```python
from build123d import *

# Parameters (mm, degrees)
SKETCH_R              = 9.5
PAD_DEPTH             = 0.4
POLARPATTERN_COUNT    = 6
PAD001_DEPTH          = 25
POLARPATTERN001_COUNT = 6
SKETCH002_R           = 9.5
POCKET_DEPTH          = 2
POLARPATTERN002_COUNT = 6
SKETCH003_R           = 1.5
PAD002_DEPTH          = 25


with BuildPart() as part:
    # Sketch → Pad (new body, symmetric)
    with BuildSketch(Plane.XZ):
        with BuildLine():
            Line((0, 0), (57, 0))
            Line((57, 0), (57, 25))
            Line((57, 25), (0, 25))
            Line((0, 25), (0, 22))
            ThreePointArc((0, 3), (9.5, 12.5), (0, 22))
            Line((0, 3), (0, 0))
        make_face()
        with Locations((22, 12.5)):
            Circle(SKETCH_R, mode=Mode.SUBTRACT)
        with Locations((44, 12.5)):
            Circle(SKETCH_R, mode=Mode.SUBTRACT)
    pad = extrude(amount=PAD_DEPTH, both=True)

    # PolarPattern: Pad ×6 about axis
    polarpattern_axis = Axis((0, 0, 0), (0, 0, 1))
    for i in range(1, POLARPATTERN_COUNT):
        add(pad.rotate(polarpattern_axis, i * 360 / POLARPATTERN_COUNT))

    # Sketch001 (on Face55 of PolarPattern) → Pad001 (join)
    with BuildSketch(Plane(origin=(0, 0, 25), x_dir=(-1, 0, 0), z_dir=(0, 0, 1))):
        Polygon((-28.15359, 49.563448), (28.15359, 49.563448), (27.69171, 48.763448), (-27.69171, 48.763448), align=None)
    pad001 = extrude(amount=-PAD001_DEPTH)

    # PolarPattern001: Pad001 ×6 about axis
    polarpattern001_axis = Axis((0, 0, 25), (0, 0, 1))
    for i in range(1, POLARPATTERN001_COUNT):
        add(pad001.rotate(polarpattern001_axis, i * 360 / POLARPATTERN001_COUNT))

    # Sketch002 (on Face59 of Pad001) → Pocket (cut)
    with BuildSketch(Plane.XZ.offset(49.563448)):
        with Locations((-12.5, 12.5)):
            Circle(SKETCH002_R)
        with Locations((12.5, 12.5)):
            Circle(SKETCH002_R)
    pocket = extrude(amount=-POCKET_DEPTH, mode=Mode.SUBTRACT)

    # PolarPattern002: Pocket ×6 about axis
    polarpattern002_axis = Axis((0, 0, 0), (0, 0, 1))
    for i in range(1, POLARPATTERN002_COUNT):
        add(pocket.rotate(polarpattern002_axis, i * 360 / POLARPATTERN002_COUNT), mode=Mode.SUBTRACT)

    # Sketch003 (on Face81 of PolarPattern002) → Pad002 (join)
    with BuildSketch(Plane(origin=(0, 0, 25), x_dir=(-1, 0, 0), z_dir=(0, 0, 1))):
        Circle(SKETCH003_R)
    extrude(amount=-PAD002_DEPTH)


solid = part.part
```
Input: part model. Units: mm. Frame: model coordinates. A direction names the side the tool comes from. Give positions to 0.01 mm unless a question says otherwise; leave off trailing zeros. Return JSON: item names as keys, results as strings.
1) Line query: L1, parallel to Z at x = 44, y = 0; L2, parallel to Y at x = 1, z = 3.5; L3, parallel to Y at x = 27, z = 24. Output: solid intervals per line, ascending. Write a range as [from, to].
Taken from the geometry:
{"L1": "z = [0, 3], [22, 25]", "L2": "y = [-49.56, -48.76], [-1.12, 1.12], [48.76, 49.56]", "L3": "y = [-49.56, -48.76], [-47.57, -45.97], [-0.4, 0.4], [45.97, 47.57], [48.76, 49.56]"}
2) Section query A-A on x = -39. Count the separate pieces of the cut face and the enclosed holes in it, and give its area (3 significant figures).
Taken from the geometry:
{"separate pieces": "6", "enclosed holes": "0", "area": "36.9 mm2"}
3) Contact query for flat-ended pins moving along their axis: pin 1 (10 mm diameter, centred on y = 14, z = 6.5, fed in from +X); pin 2 (11.5 mm diameter, centred on x = 12.5, z = 12.5, fed in from -Y); pin 3 (10 mm diameter, centred on y = 23, z = 3.5, fed in from -X). Output: stop coordinate, or through.
Taken from the geometry:
{"pin 1": "stops at x = 51.82", "pin 2": "stops at y = -30.59", "pin 3": "stops at x = -46.84"}
4) Mould query, pull axis X, two halves, no side actions, for faces 1 (the face through (16.878, -30.033, 15.453)), 2 (the face through (-42.73, -25.12, 12.68)), 3 (the face through (0, 49.563, 13)). Classes: released by +X, released by -X, zero draft, split by the parting line, or undercut.
Taken from the geometry:
{"face 1": "undercut", "face 2": "released by -X", "face 3": "zero draft"}
5) Access query for faces 4 (the face through (9.5, 0.01, 12.69)), 5 (the face through (-5.5, 49.17, 18.92)), 6 (the face through (42.037, -24.717, 12.675)). Directions: +Z, -Z, +X, -X, +Y, -Y. A direction counts if a zero-diameter tool reaches every point of the face in a straight line with its end or side. Return the directions, or none.
Taken from the geometry:
{"face 4": "none", "face 5": "+Y", "face 6": "+Z, -Z"}
